Geometry: final body of the model. Coordinates: model frame, mm. A direction names the side the tool comes from. Round coordinates to 2 decimals unless told otherwise and drop trailing zeros. Order: outer loops, then holes, each group sorted by start corner. A loop starts at its lowest first (then second) coordinate and runs counter-clockwise, first axis right, second up. Notation, with made-up numbers: M 5.25,45 L 48.25,45 A5 cw 48.25,54 Z; hole C 12.5,19 d9. An arc over 180 degrees is marked long. Return JSON: item names as keys, results as strings. Group by question number.
Q1. Cut plane D-D on x = -7. Output: boundary loops of the cut face in (y, z).
Q2. Cut plane B-B on x = -43. Output: boundary loops of the cut face in (y, z), and give its area (3 significant figures).
Q3. Contact query for flat-ended pins moving along their axis: pin 1 (5 mm diameter, centred on x = -7, y = -6.5, fed in from -Z); pin 2 (10 mm diameter, centred on x = -10, y = -36.5, fed in from +Z); pin 3 (15.5 mm diameter, centred on y = 0, z = -42, fed in from +X); pin 4 (1.5 mm diameter, centred on x = -28, z = 24.5, fed in from +Y). Output: stop coordinate, or through.
Q4. Mould query, pull axis X, two halves, no side actions, for faces 1 (the face through (-35.993, 2.103, 45.677)), 2 (the face through (-40.1, -5, 39)), 3 (the face through (-4.2, -24.3, -10.1)), 4 (the face through (-65, -9, 25)). Classes: released by +X, released by -X, zero draft, split by the parting line, or undercut.
Q5. Ray query, probe 1 along X at (y, z) = (18.5, 18.5); probe 2 along X at (y, z) = (-24.5, -18); probe 3 along Y at (x, z) = (-43.5, 16.5). Return the intervals inside material, ascending.
Q6. Access query for faces 5 (the face through (-45, -18, 25)), 6 (the face through (-11.595, -15.821, -20.633)), 7 (the face through (-3.085, -24.397, 12.69)). Directions: +Z, -Z, +X, -X, +Y, -Y. A direction counts if a zero-diameter tool reaches every point of the face in a straight line with its end or side. Return the directions, or none.
Q7. Cut plane A-A on y = 39. Output: boundary loops of the cut face in (x, z).
```python
from build123d import *

# Parameters (mm, degrees)
SKETCH7_R          = 72
CUT_EXTRUDE1_DEPTH = 13


with BuildPart() as part:
    # Sketch1 → Revolve1 (revolve)
    with BuildSketch(Plane.XY, mode=Mode.PRIVATE) as revolve1_sk:
        Polygon((-65, 0), (-65, 30), (-45, 30), (-45, 47), (-32, 47), (-32, 30), (0, 30), (0, 0), align=None)
    revolve(revolve1_sk.sketch.rotate(Axis((0, 0, 0), (-1, 0, 0)), 180), axis=Axis((0, 0, 0), (-1, 0, 0)))

    # Sketch2 → Cut-Revolve1 (revolve, cut)
    with BuildSketch(Plane.XY, mode=Mode.PRIVATE) as cut_revolve1_sk:
        Polygon((-65, 0), (-65, 26), (-63, 26), (-63, 27.5), (-60.8, 27.5), (-60.8, 26), (-45.8, 26), (-45.8, 22.5), (-19.2, 22.5), (-19.2, 26), (-4.2, 26), (-4.2, 27.5), (-2, 27.5), (-2, 26), (0, 26), (0, 0), align=None)
    revolve(cut_revolve1_sk.sketch.rotate(Axis((0, 0, 0), (-1, 0, 0)), 270), axis=Axis((0, 0, 0), (-1, 0, 0)), mode=Mode.SUBTRACT)

    # Sketch3 → Cut-Revolve2 (revolve, cut)
    with BuildSketch(Plane.XY, mode=Mode.PRIVATE) as cut_revolve2_sk:
        Polygon((-45, 39), (-45, 43.5), (-40.1, 43.5), (-40.1, 46), (-32, 46), (-32, 39), align=None)
    revolve(cut_revolve2_sk.sketch.rotate(Axis((-32, 39, 0), (-1, 0, 0)), 270), axis=Axis((-32, 39, 0), (-1, 0, 0)), mode=Mode.SUBTRACT)

    # Sketch4 → Cut-Revolve3 (revolve, cut)
    with BuildSketch(Plane.XY.offset(39), mode=Mode.PRIVATE) as cut_revolve3_sk:
        Polygon((-45, 0), (-45, 4.5), (-40.1, 4.5), (-40.1, 7), (-32, 7), (-32, 0), align=None)
    revolve(cut_revolve3_sk.sketch.rotate(Axis((-32, 0, 39), (-1, 0, 0)), 270), axis=Axis((-32, 0, 39), (-1, 0, 0)), mode=Mode.SUBTRACT)

    # Sketch5 → Cut-Revolve4 (revolve, cut)
    with BuildSketch(Plane.XY, mode=Mode.PRIVATE) as cut_revolve4_sk:
        Polygon((-45, -39), (-45, -34.5), (-40.1, -34.5), (-40.1, -32), (-32, -32), (-32, -39), align=None)
    revolve(cut_revolve4_sk.sketch.rotate(Axis((-32, -39, 0), (-1, 0, 0)), 270), axis=Axis((-32, -39, 0), (-1, 0, 0)), mode=Mode.SUBTRACT)

    # Sketch6 → Cut-Revolve5 (revolve, cut)
    with BuildSketch(Plane.XY.offset(-39), mode=Mode.PRIVATE) as cut_revolve5_sk:
        Polygon((-45, 0), (-45, 4.5), (-40.1, 4.5), (-40.1, 7), (-32, 7), (-32, 0), align=None)
    revolve(cut_revolve5_sk.sketch.rotate(Axis((-32, 0, -39), (-1, 0, 0)), 270), axis=Axis((-32, 0, -39), (-1, 0, 0)), mode=Mode.SUBTRACT)

    # Sketch7 → Cut-Extrude1 (cut)
    with BuildSketch(Plane(origin=(-32, 0, 0), x_dir=(0, 0, -1), z_dir=(1, 0, 0))):
        Circle(SKETCH7_R)
        Polygon((-50.911688245, 0), (0, -50.911688245), (50.911688245, 0), (0, 50.911688245), align=None, mode=Mode.SUBTRACT)
    extrude(amount=-CUT_EXTRUDE1_DEPTH, mode=Mode.SUBTRACT)


solid = part.part
```
Result sheet:
{
 "1": {"outline": "C 0,0 d60; hole C 0,0 d52"},
 "2": {"outline": "M -46.82,-4.09 L -4.09,-46.82 A47 ccw 4.09,-46.82 L 46.82,-4.09 A47 ccw 46.82,4.09 L 4.09,46.82 A47 ccw -4.09,46.82 L -46.82,4.09 A47 ccw Z; hole C -39,0 d9; hole C 0,0 d45; hole C 0,-39 d9; hole C 0,39 d9; hole C 39,0 d9", "area": "3,280 mm²"},
 "3": {"pin 1": "stops at z = -29.73", "pin 2": "passes through", "pin 3": "stops at x = -32", "pin 4": "stops at y = 18.33"},
 "4": {"face 1": "zero draft", "face 2": "released by +X", "face 3": "undercut", "face 4": "released by -X"},
 "5": {"probe 1": "x = -65 to -63, -60.8 to -4.2, -2 to 0", "probe 2": "x = -45 to -32", "probe 3": "y = -34.41 to -15.3, 15.3 to 34.41"},
 "6": {"face 5": "-X", "face 6": "+X", "face 7": "none"},
 "7": {"outline": "M -45,-11.91 L -32,-11.91 L -32,-7 L -40.1,-7 L -40.1,-4.5 L -45,-4.5 Z; M -45,4.5 L -40.1,4.5 L -40.1,7 L -32,7 L -32,11.91 L -45,11.91 Z"}
}
